Input: part model. Units: mm. Frame: model coordinates. Face numbers are marked on the shaded views. A direction names the side the tool comes from. Coordinates: 2 decimals unless noted, no trailing zeros. Loops run counter-clockwise (first coordinate to the right, second up) from the corner with the lowest first, then second, coordinate; pieces in that order, holes last. Notation, with made-up numbers: (64.5, -9.75) - (72.5, -9.75) arc R27 cw to (72.5, 8.25) - close; hole circle Ø11 at (72, -15). An arc over 180 degrees is marked (long way). Write item = value, one per line. Start each with the question number.
from build123d import *

# Parameters (mm, degrees)
F0_W     = 31.75
F0_H     = 38.1
F1_DEPTH = 50.8
F3_DEPTH = 50.801
F4_W     = 25.4
F4_H     = 18.65923
F5_DEPTH = 25.4


with BuildPart() as f1:
    # F0 (on Right) → F1 (new body)
    with BuildSketch(Plane.YZ):
        with Locations((-43.14976, 19.05)):
            Rectangle(F0_W, F0_H)
    extrude(amount=F1_DEPTH)

    # F2 (on face) → F3 (cut, through all)
    with BuildSketch(Plane.YZ.offset(50.8)):
        with BuildLine():
            Line((-59.02476, 38.1), (-59.02476, 12.7))
            ThreePointArc((-59.02476, 12.7), (-39.27704, 18.35228), (-33.62476, 38.1))
            Line((-33.62476, 38.1), (-59.02476, 38.1))
        make_face()
    extrude(amount=-F3_DEPTH, mode=Mode.SUBTRACT)

    # F4 (on face) → F5 (cut)
    with BuildSketch(Plane(origin=(0, -27.27476, 0), x_dir=(-1, 0, 0), z_dir=(0, 1, 0))):
        with Locations((-25.4, 28.770385)):
            Rectangle(F4_W, F4_H)
    extrude(amount=-F5_DEPTH, mode=Mode.SUBTRACT)


solid = f1.part
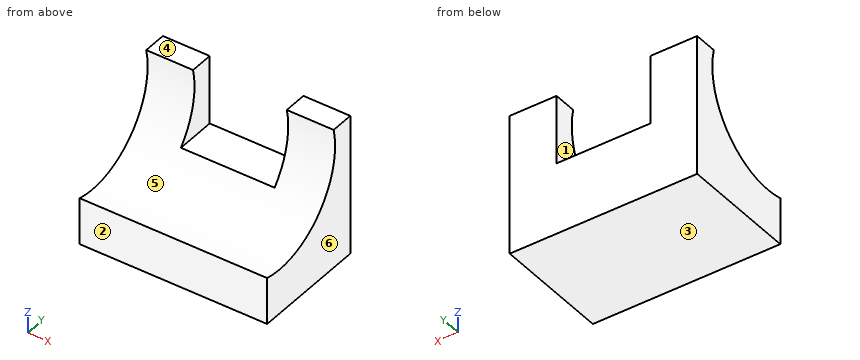
Item 1: Cut plane B-B on y = -30.5. Return loops of the section in (x, z).
Item 2: Cut plane A-A on z = 23. Return loops of the section in (x, y).
Item 3: Pin query (flat end, axial travel): pin 1 (10 mm diameter, centred on x = 6.5, y = -48.5, fed in from +Z); pin 2 (1 mm diameter, centred on x = 8, z = 33, fed in from -Y); pin 3 (2 mm diameter, centred on x = 11, y = -48.5, fed in from +Z). Return the tip coordinate at first contact, or that it passes through.
Item 4: Ray query, line 1 (X direction, y = -33, z = 31); line 2 (Y direction, x = 10, z = 33.5); line 3 (Z direction, x = 22, y = -33.5). Return the intervals inside material, ascending.
Item 5: Pull-direction query (Z, two-part tool) for the marked faces 3, 4, 5 and 6; classes: pulls with the +Z half, pulls with the -Z half, needs draft (parallel to the pull), parting line crosses it, or undercut.
Item 6: Access query for the marked faces 1 and 2. Directions: +Z, -Z, +X, -X, +Y, -Y. A direction counts if a zero-diameter tool reaches every point of the face in a straight line with its end or side. Return the directions, or none.
Item 7: Cut plane C-C on x = 37. Return loops of the section in (y, z).
Item 8: Cut plane D-D on z = 27.5. Return loops of the section in (x, y), plus the area to 3 significant figures.
Recorded:
q1.outline = (0, 0) - (50.8, 0) - (50.8, 38.1) - (38.1, 38.1) - (38.1, 19.44) - (12.7, 19.44) - (12.7, 38.1) - (0, 38.1) - close
q2.outline = (0, -35.76) - (12.7, -35.76) - (12.7, -27.27) - (0, -27.27) - close; (38.1, -35.76) - (50.8, -35.76) - (50.8, -27.27) - (38.1, -27.27) - close
q3.pin_1 = 15.08
q3.pin_2 = -33.09
q3.pin_3 = 13.26
q4.line_1 = 0 to 12.7, 38.1 to 50.8
q4.line_2 = -33.08 to -27.27
q4.line_3 = 0 to 19.44
q5.face_3 = pulls with the -Z half
q5.face_4 = pulls with the +Z half
q5.face_5 = undercut
q5.face_6 = needs draft
q6.face_1 = +Z, +Y, -Y
q6.face_2 = +Z, -Z, +X, -X, -Y
q7.outline = (-59.02, 0) - (-27.27, 0) - (-27.27, 19.44) - (-38.26, 19.44) arc R21.17 cw to (-59.02, 12.7) - close
q8.outline = (0, -33.89) - (12.7, -33.89) - (12.7, -27.27) - (0, -27.27) - close; (38.1, -33.89) - (50.8, -33.89) - (50.8, -27.27) - (38.1, -27.27) - close
q8.area = 168 mm²
